CAD build for the part. Positions are in the model's coordinates, mm. A direction names the side the tool comes from. Round coordinates to 2 decimals unless told otherwise and drop trailing zeros. Write each loop counter-clockwise with the first axis right and the second up, starting at its lowest first coordinate (ties: lowest second). Pieces come first, ordered by that corner, then holes. Notation, with made-up numbers: (39.5, 53) -> (50.5, 53) arc R16 ccw to (50.5, 72) -> close; hole circle Ø3 at (40.5, -31). An arc over 180 degrees is marked (long way). Answer in a Markdown table with one row per item. Add a question column.
Autodesk Fusion 360 part; units mm, degrees
sketch "Sketch1" plane through (0, 0, 0) normal (0, 0, 1) x (1, 0, 0) in component "Component"
  line L0 (0, 23.2) -> (86.2, 23.2) construction
  line L1 (86.2, 23.2) -> (86.2, 0) construction
  line L2 (86.2, 0) -> (0, 0) construction
  line L3 (0, 0) -> (0, 23.2) construction
  line L4 (86.2, 20.3) -> (82.8, 20.3)
  line L5 (82.8, 20.3) -> (82.8, 23.2)
  line L6 (82.8, 23.2) -> (63.2045, 23.2)
  line L7 (63.3, 23.2) -> (63.3, 20.8)
  line L8 (63.3, 20.8) -> (61.1, 20.8)
  line L9 (61.1, 20.8) -> (61.1, 23.2)
  line L10 (61.1, 23.2) -> (49.1, 23.2)
  line L11 (49.1, 23.2) -> (49.1, 18.6)
  line L12 (49.1, 18.6) -> (46.9, 18.6)
  line L13 (46.9, 18.6) -> (46.9, 23.2)
  line L14 (46.9, 23.2) -> (10, 23.2)
  line L15 (10, 23.2) -> (0, 18.2)
  line L16 (0, 18.2) -> (0, 5)
  line L17 (0, 5) -> (10, 0)
  line L18 (10, 0) -> (45, 0)
  line L19 (45, 0) -> (45, 2.6)
  line L20 (45, 2.6) -> (47.2, 2.6)
  line L21 (47.2, 2.6) -> (47.2, 0)
  line L22 (47.2, 0) -> (86.2, 0)
  line L23 (86.2, 0) -> (86.2, 20.3)
  circle A0 centre (25.2, 5) radius 2.5
  line L24 (78.4, 10.9318) -> (78.4, 4.2318)
  arc A1 (78.4, 4.2318) -> (81.9, 4.2318) centre (80.15, 4.2318) ccw
  line L25 (81.9, 4.2318) -> (81.9, 10.9318)
  arc A2 (81.9, 10.9318) -> (78.4, 10.9318) centre (80.15, 10.9318) ccw
  line L26 (55.1, 12) -> (54.6, 12)
  line L27 (54.6, 12) -> (54.6, 11)
  line L28 (54.6, 11) -> (55.1, 11)
  line L29 (55.1, 11) -> (55.1, 12)
  line L30 (79, 18.2) -> (79.5, 18.2)
  line L31 (79.5, 18.2) -> (79.5, 17.7)
  line L32 (79.5, 17.7) -> (79, 17.7)
  line L33 (79, 17.7) -> (79, 18.2)
  dimension "d1" = 86.2
  dimension "d2" = 23.2
  dimension "d3" = 2.2
  dimension "d4" = 2.2
  dimension "d5" = 4.6
  dimension "d6" = 2.4
  dimension "d7" = 2.2
  dimension "d8" = 2.6
  dimension "d9" = 3.4
  dimension "d10" = 2.9
  dimension "d11" = 10
  dimension "d12" = 5
  dimension "d13" = 25.2
  dimension "d14" = 5
  dimension "d15" = 5
  dimension "d16" = 45
  dimension "d17" = 46.9
  dimension "d18" = 61.1
  dimension "d19" = 6.7
  dimension "d20" = 4.3
  dimension "d21" = 4.2318
  dimension "d22" = 1.75
  dimension "d23" = 0.5
  dimension "d24" = 55.1
  dimension "d25" = 1
  dimension "d26" = 12
  dimension "d27" = 0.5
  dimension "d28" = 0.5
  dimension "d29" = 79.5
  dimension "d30" = 5
extrude "Extrude1" add sketch "Sketch1" along normal blind 1.6 in component "Component"
component "Component" placed x (1, 0, 0) y (0, 1, 0) z (0, 0, 1) at (0, 0, 0)
Item 1: Saw through at C-C on z = 0.8. Count the separate pieces of the cut face and the enclosed holes in it, then the cut area to 3 significant figures.
Item 2: Saw through at A-A on x = 25.2. Give the cut face in (y, z), then the cut area to 3 significant figures.
Item 3: Two-plate mould, pull along X, no slides. Class faces 5 (the flat face through (5.07, 20.735, 0.789)), 6 (the cylindrical face through (80.11, 12.68, 0.79)), 7 (the flat face through (66, 0, 1)), 8 (the flat face through (82.8, 22, 1)): +X half, -X half, draft (parallel to the pull), parting line (faces both ways), or undercut.
Item 4: Pin check, flat tips, straight feed: pin 1 (0.5 mm diameter, centred on y = 21.5, z = 0.5, fed in from -X); pin 2 (0.8 mm diameter, centred on x = 48, z = 0.5, fed in from +Y); pin 3 (3 mm diameter, centred on x = 25.2, y = 5, fed in from +Z); pin 4 (0.8 mm diameter, centred on x = 46.5, z = 1, fed in from -Y). Stop position of each tip, or through.
Item 5: Tool access for faces 1 (the flat face through (81.9, 8, 1)), 2 (the flat face through (48, 18.6, 1)), 3 (the flat face through (45, 1, 1)), 4 (the flat face through (85, 20.3, 1)): list every direction of +Z, -Z, +X, -X, +Y, -Y with a clear straight run to the whole face (end or side of a thin tool).
Item 6: Saw through at B-B on y = 21.75. Give the cut face in (x, z).
Item 7: Drill centre lines: probe 1 along X at (y, z) = (10.75, 1.3); probe 2 along Y at (x, z) = (25.2, 0.4); probe 3 along X at (y, z) = (17.75, 0.3). Where is each one in solid material? Low to high.
Recorded:
| question | item | result |
|---|---|---|
| 1 | separate pieces | 1 |
| 1 | enclosed holes | 4 |
| 1 | area | 1,870 mm2 |
| 2 | outline | (0, 0) -> (2.5, 0) -> (2.5, 1.6) -> (0, 1.6) -> close; (7.5, 0) -> (23.2, 0) -> (23.2, 1.6) -> (7.5, 1.6) -> close |
| 2 | area | 29.1 mm2 |
| 3 | face 5 | -X half |
| 3 | face 6 | undercut |
| 3 | face 7 | draft |
| 3 | face 8 | +X half |
| 4 | pin 1 | x = 6.1 |
| 4 | pin 2 | y = 18.6 |
| 4 | pin 3 | through |
| 4 | pin 4 | y = 2.6 |
| 5 | face 1 | +Z, -Z |
| 5 | face 2 | +Z, -Z, +Y |
| 5 | face 3 | +Z, -Z, -Y |
| 5 | face 4 | +Z, -Z, +X, +Y |
| 6 | outline | (7.1, 0) -> (46.9, 0) -> (46.9, 1.6) -> (7.1, 1.6) -> close; (49.1, 0) -> (61.1, 0) -> (61.1, 1.6) -> (49.1, 1.6) -> close; (63.3, 0) -> (82.8, 0) -> (82.8, 1.6) -> (63.3, 1.6) -> close |
| 7 | probe 1 | 0 to 78.4, 81.9 to 86.2 |
| 7 | probe 2 | 0 to 2.5, 7.5 to 23.2 |
| 7 | probe 3 | 0 to 79, 79.5 to 86.2 |
